from build123d import *

# Parameters (mm, degrees)
F0_R     = 46
F0_R_2   = 40
F1_DEPTH = 13
F3_R     = 5
F4_DEPTH = 10
F5_SIZE2 = 3.2153903092
F5_SIZE  = 12
F6_SIZE2 = 5
F6_SIZE  = 1


with BuildPart() as f1:
    # F0 (on Top) → F1 (new body)
    with BuildSketch(Plane.XY):
        Circle(F0_R)
        Circle(F0_R_2, mode=Mode.SUBTRACT)
    extrude(amount=F1_DEPTH)

    # F3 (on offset) → F4 (join)
    with BuildSketch(Plane.XZ.offset(44.5)):
        with Locations((0, 6.839911745)):
            Circle(F3_R)
    extrude(amount=F4_DEPTH)

    # F5
    f5_edges = [f1.edges().sort_by_distance(p)[0] for p in [
        (-40, 0, 13),
    ]]
    f5_side = f1.faces().sort_by_distance((-40, 0, 6.5))[0]
    chamfer(f5_edges, length=F5_SIZE, length2=F5_SIZE2, reference=f5_side)

    # F6
    f6_edges = [f1.edges().sort_by_distance(p)[0] for p in [
        (-5, -54.5, 6.839912),
    ]]
    f6_side = f1.faces().sort_by_distance((0, -54.5, 6.839912))[0]
    chamfer(f6_edges, length=F6_SIZE, length2=F6_SIZE2, reference=f6_side)


solid = f1.part
Verification items for the finished model (mm, model axes). A direction names the side the tool comes from. Give positions to 0.01 mm unless a question says otherwise; leave off trailing zeros. Loops run counter-clockwise (first coordinate to the right, second up) from the corner with the lowest first, then second, coordinate; pieces in that order, holes last.
1) Thickness scan on line 1 along Y through (x, z) = (0, 0.65); line 2 along X through (y, z) = (39, 10.5); line 3 along X through (y, z) = (20.5, 2.25). Record the ranges inside material, lowest first.
2) Sectioned sample at A-A, the plane x = 0. Enter the section's corners in (y, z).
3) Set-up check for faces 1 (the flat face through (-14, 38, 0)), 2 (the cylindrical face through (-4.995, -47.587, 7.06)): record each of +Z, -Z, +X, -X, +Y, -Y from which the full face is reachable in a straight line by a thin tool's end or side.
4) Sectioned sample at B-B, the plane y = 0. Enter the section's corners in (x, z), then the cut area to 3 significant figures.
5) Depth check by flat-ended pin: pin 1 Ø6 at (x, z) = (-2.5, 9) entering from +Y; pin 2 Ø1 at (y, z) = (22, 8) entering from -X; pin 3 Ø1.5 at (y, z) = (13.5, 4) entering from +X. Enter the tip coordinate at first touch or a pass-through.
6) Draft check along Y on faces 3 (the flat face through (-13.84, 41.1, 13)), 4 (the flat face through (0, -54.5, 7)), 5 (the cylindrical face through (-8.67, -39.05, 0.49)). Enter one of: pulls with the +Y half, pulls with the -Y half, needs draft (parallel to the pull), parting line crosses it, or undercut.
Answers:
1. line 1: y = -46 to -40, 40 to 46
1. line 2: x = -24.39 to -17, 17 to 24.39
1. line 3: x = -41.18 to -34.74, 34.74 to 41.18
2. outline: (-54.5, 2.84) - (-49.5, 1.84) - (-46, 1.84) - (-46, 0) - (-40, 0) - (-40, 1) - (-43.22, 13) - (-46, 13) - (-46, 11.84) - (-49.5, 11.84) - (-54.5, 10.84) - close; (40, 0) - (46, 0) - (46, 13) - (43.22, 13) - (40, 1) - close
3. face 1: -Z, +X, -X, +Y, -Y
3. face 2: -Y
4. outline: (-46, 0) - (-40, 0) - (-40, 1) - (-43.22, 13) - (-46, 13) - close; (40, 0) - (46, 0) - (46, 13) - (43.22, 13) - (40, 1) - close
4. area: 117 mm2
5. pin 1: stops at y = 46
5. pin 2: stops at x = -40.67
5. pin 3: stops at x = 44.2
6. face 3: needs draft
6. face 4: pulls with the -Y half
6. face 5: undercut
